Geometry: see drawing. Coordinates: mm, zero at the bounding-box minimum. A direction names the side the tool comes from. Round coordinates to 2 decimals unless told otherwise and drop trailing zeros. Loops run counter-clockwise (first coordinate to the right, second up) from the corner with the lowest first, then second, coordinate; pieces in that order, holes last. Notation, with made-up numbers: M 84,-8 L 114,-8 A16 ccw 114,-2 Z; hole C 9,-29 d6. An arc over 180 degrees is marked long. Answer as a JSON object with one key per item and string values.
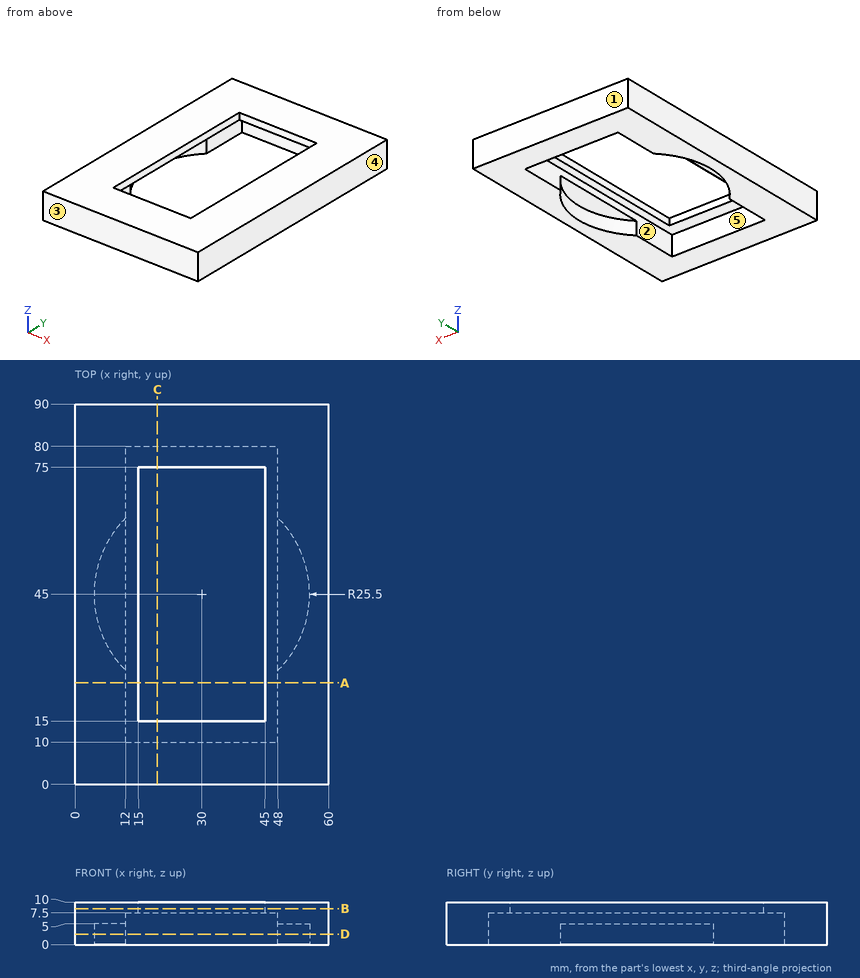
1) Section query B-B (z = 8.5). Return the cut outline in (x, y), and give its area (3 significant figures).
Results:
{"outline": "M 0,0 L 60,0 L 60,90 L 0,90 Z; hole M 15,15 L 45,15 L 45,75 L 15,75 Z", "area": "3,600 mm2"}
2) Section query A-A (y = 24). Return the cut outline in (x, z), and give its area (3 significant figures).
Results:
{"outline": "M 0,0 L 12,0 L 12,7.5 L 15,7.5 L 15,10 L 0,10 Z; M 45,7.5 L 48,7.5 L 48,0 L 60,0 L 60,10 L 45,10 Z", "area": "255 mm2"}
3) Pull-direction query (X, two-part tool) for the marked faces 3, 4 and 5; classes: +X half, -X half, draft (parallel to the pull), parting line (faces both ways), or undercut.
Results:
{"face 3": "draft", "face 4": "+X half", "face 5": "undercut"}
4) Section query D-D (z = 2.5). Return the cut outline in (x, y).
Results:
{"outline": "M 0,0 L 60,0 L 60,90 L 0,90 Z; hole M 12,10 L 48,10 L 48,26.94 A25.5 ccw 48,63.06 L 48,80 L 12,80 L 12,63.06 A25.5 ccw 12,26.94 Z"}
5) Ray query, line 1 (X direction, y = 67.5, z = 3.5); line 2 (Y direction, x = 40.5, z = 7.25); line 3 (X direction, y = 52, z = 9.25). Return the intervals inside material, ascending.
Results:
{"line 1": "0 to 12, 48 to 60", "line 2": "0 to 10, 80 to 90", "line 3": "0 to 15, 45 to 60"}
6) Section query C-C (x = 19.5). Return the cut outline in (y, z), and give its area (3 significant figures).
Results:
{"outline": "M 0,0 L 10,0 L 10,7.5 L 15,7.5 L 15,10 L 0,10 Z; M 75,7.5 L 80,7.5 L 80,0 L 90,0 L 90,10 L 75,10 Z", "area": "225 mm2"}
7) Pin query (flat end, axial travel): P1, Ø4, axis at x = 51, y = 37, coming from the -Z side; P2, Ø18, axis at x = 29.5, y = 48.5, coming from the -Z side. Return the tip coordinate at first contact, or that it passes through.
Results:
{"P1": "z = 5", "P2": "through"}
8) Reachability of the marked faces 1 and 2 from +Z, -Z, +X, -X, +Y, -Y: full face, straight path, thin tool, end or side. Return the list, or none.
Results:
{"face 1": "+Z, -Z, +X, -X, +Y", "face 2": "-Z"}
